Verification items for the finished model (mm, model axes). Face numbers are marked on the shaded views. Coordinates: 2 decimals unless noted, no trailing zeros. Write each loop counter-clockwise with the first axis right and the second up, starting at its lowest first coordinate (ties: lowest second). Pieces come first, ordered by that corner, then holes. Notation, with made-up numbers: (-1.5, -3.75) -> (2.5, -3.75) arc R20 ccw to (2.5, 22.25) -> close; hole circle Ø8 at (-40, 37). An arc over 180 degrees is marked (long way). Use CSV: the item, a comma, the result in double quotes.
```python
from build123d import *

# Parameters (mm, degrees)
SKETCH1_R                    = 24
SKETCH1_R_2                  = 22.8
BOSS_EXTRUDE1_DEPTH          = 2.5
BOSS_EXTRUDE5_START          = -2.5
BOSS_EXTRUDE5_DEPTH          = 1.5
CIRPATTERN1_COUNT            = 4
SKETCH2_R                    = 27
BOSS_EXTRUDE2_DEPTH          = 2
SKETCH3_R                    = 7.1
CUT_EXTRUDE1_DEPTH           = 39.448016854
SKETCH4_R                    = 8.3
SKETCH4_R_2                  = 7.1
BOSS_EXTRUDE3_DEPTH          = 2.5
BOSS_EXTRUDE4_START          = -1.5
SKETCH5_R                    = 8.3
SKETCH5_R_2                  = 6.3
BOSS_EXTRUDE4_DEPTH          = 1.5
CUT_EXTRUDE2_DEPTH           = 2.5
CHAMFER2_SIZE                = 2.5
CIRPATTERN2_COUNT            = 4
CHAMFER2_OF_CIRPATTERN2_SIZE = 2.5
FILLET1_R                    = 2
CHAMFER1_SIZE                = 0.5


# Some blends are built 0.0001 mm under size
with BuildPart() as part:
    # Sketch1 → Boss-Extrude1 (new body)
    with BuildSketch(Plane.XY):
        Circle(SKETCH1_R)
        Circle(SKETCH1_R_2, mode=Mode.SUBTRACT)
    extrude(amount=BOSS_EXTRUDE1_DEPTH)

    # Sketch6 → Boss-Extrude5 (add)
    with BuildSketch(Plane.XY.offset(2.5).offset(BOSS_EXTRUDE5_START)):
        with BuildLine():
            ThreePointArc((23.953079134, 1.5), (24, 0), (23.953079134, -1.5))
            ThreePointArc((23.953079134, -1.5), (24.3, 0), (23.953079134, 1.5))
        make_face()
    boss_extrude5 = extrude(amount=BOSS_EXTRUDE5_DEPTH)

    # CirPattern1: Boss-Extrude5 ×4 about axis
    cirpattern1_axis = Axis((0, 0, 0), (0, 0, 1))
    for i in range(1, CIRPATTERN1_COUNT):
        add(boss_extrude5.rotate(cirpattern1_axis, i * 360 / CIRPATTERN1_COUNT))

    # Sketch2 → Boss-Extrude2 (add)
    with BuildSketch(Plane.XY.offset(2.5)):
        Circle(SKETCH2_R)
    extrude(amount=BOSS_EXTRUDE2_DEPTH)

    # Sketch3 → Cut-Extrude1 (cut, through all)
    with BuildSketch(Plane.XY.offset(4.5)):
        Circle(SKETCH3_R)
    extrude(amount=-CUT_EXTRUDE1_DEPTH, mode=Mode.SUBTRACT)

    # Sketch4 → Boss-Extrude3 (add, through all)
    with BuildSketch(Plane(origin=(0, 0, 2.5), x_dir=(-1, 0, 0), z_dir=(0, 0, -1))):
        with Locations(Location((0, 0, 0), (0, 0, 180))):
            Circle(SKETCH4_R)
        with Locations(Location((0, 0, 0), (0, 0, 180))):
            Circle(SKETCH4_R_2, mode=Mode.SUBTRACT)
    extrude(amount=BOSS_EXTRUDE3_DEPTH)

    # Sketch5 → Boss-Extrude4 (add)
    with BuildSketch(Plane(origin=(0, 0, 0), x_dir=(-1, 0, 0), z_dir=(0, 0, -1)).offset(BOSS_EXTRUDE4_START)):
        with Locations(Location((0, 0, 0), (0, 0, 180))):
            Circle(SKETCH5_R)
        Circle(SKETCH5_R_2, mode=Mode.SUBTRACT)
    extrude(amount=BOSS_EXTRUDE4_DEPTH)

    # Sketch7 → Cut-Extrude2 (cut)
    with BuildSketch(Plane(origin=(0, 0, 0), x_dir=(-1, 0, 0), z_dir=(0, 0, -1))):
        with BuildLine():
            ThreePointArc((8.725182258, 21.064453341), (12.667001313, 18.95750716), (16.122034611, 16.122034611))
            Line((16.122034611, 16.122034611), (16.970562748, 16.970562748))
            ThreePointArc((16.970562748, 16.970562748), (13.333685592, 19.955270695), (9.184402377, 22.17310878))
            Line((9.184402377, 22.17310878), (8.725182258, 21.064453341))
        make_face()
        with BuildLine():
            Line((16.970562748, 16.970562748), (16.122034611, 16.122034611))
            ThreePointArc((16.122034611, 16.122034611), (18.95750716, 12.667001313), (21.064453341, 8.725182258))
            Line((21.064453341, 8.725182258), (22.17310878, 9.184402377))
            ThreePointArc((22.17310878, 9.184402377), (19.955270695, 13.333685592), (16.970562748, 16.970562748))
        make_face()
    cut_extrude2 = extrude(amount=-CUT_EXTRUDE2_DEPTH, mode=Mode.SUBTRACT)

    # Chamfer2
    chamfer2_edges = [part.edges().sort_by_distance(p)[0] for p in [
        (-21.618781061, 8.954792317, 2.5),
        (-8.954792317, 21.618781061, 2.5),
    ]]
    chamfer(chamfer2_edges, length=CHAMFER2_SIZE - 0.0001)  # a hair under: the kernel refuses the full size

    # CirPattern2: Cut-Extrude2 ×4 about axis
    cirpattern2_axis = Axis((0, 0, 0), (0, 0, 1))
    for i in range(1, CIRPATTERN2_COUNT):
        add(cut_extrude2.rotate(cirpattern2_axis, i * 360 / CIRPATTERN2_COUNT), mode=Mode.SUBTRACT)

    # Chamfer2 of CirPattern2
    chamfer2_of_cirpattern2_edges = [part.edges().sort_by_distance(p)[0] for p in [
        (-8.954792317, -21.618781061, 2.5),
        (-21.618781061, -8.954792317, 2.5),
        (21.618781061, -8.954792317, 2.5),
        (8.954792317, -21.618781061, 2.5),
        (8.954792317, 21.618781061, 2.5),
        (21.618781061, 8.954792317, 2.5),
    ]]
    chamfer(chamfer2_of_cirpattern2_edges, length=CHAMFER2_OF_CIRPATTERN2_SIZE - 0.0001)  # a hair under: the kernel refuses the full size

    # Fillet1
    # the kernel refuses this fillet: 2 mm, written as the material it adds along each edge
    with BuildSketch(Plane(origin=(0, 0, 2.5), x_dir=(1, 0, 0), z_dir=(0, 1, 0))) as fillet1_piece_1:
        with BuildLine():
            CenterArc((8.3 + FILLET1_R, FILLET1_R), FILLET1_R, 180, 90)
            Line((8.3, FILLET1_R), (8.3, 0))
            Line((8.3, 0), (8.3 + FILLET1_R, 0))
        make_face()
    revolve(axis=Axis((0, 0, 2.5), (0, 0, -1)))
    with BuildSketch(Plane(origin=(0, 0, 2.5), x_dir=(0.6608111736340745, -0.7505521919229581, 0), z_dir=(0.7505521919229581, 0.6608111736340745, 0))) as fillet1_piece_2_section:
        with BuildLine():
            CenterArc((22.8 - FILLET1_R, FILLET1_R), FILLET1_R, 270, 90)
            Line((22.8, FILLET1_R), (22.8, 0))
            Line((22.8, 0), (22.8 - FILLET1_R, 0))
        make_face()
    fillet1_piece_2 = revolve(axis=Axis((0, 0, 2.5), (0, 0, -1)), revolution_arc=82.723533759, mode=Mode.PRIVATE)
    fillet1_piece_2 = split(fillet1_piece_2, bisect_by=Plane(origin=(-4.823831946, -20.235955974, -3.287225486), z_dir=(0.653281482438186, -0.27059805007310406, 0.7071067811865476)), keep=Keep.TOP, mode=Mode.PRIVATE)
    fillet1_piece_2 = split(fillet1_piece_2, bisect_by=Plane(origin=(4.823831946, -20.235955974, -3.287225486), z_dir=(-0.6532814824381898, -0.2705980500730944, 0.7071067811865478)), keep=Keep.TOP, mode=Mode.PRIVATE)
    add(fillet1_piece_2)
    with BuildSketch(Plane(origin=(0, 0, 2.5), x_dir=(0.7505521919229583, 0.6608111736340745, 0), z_dir=(-0.6608111736340745, 0.7505521919229583, 0))) as fillet1_piece_3_section:
        with BuildLine():
            CenterArc((22.8 - FILLET1_R, FILLET1_R), FILLET1_R, 270, 90)
            Line((22.8, FILLET1_R), (22.8, 0))
            Line((22.8, 0), (22.8 - FILLET1_R, 0))
        make_face()
    fillet1_piece_3 = revolve(axis=Axis((0, 0, 2.5), (0, 0, -1)), revolution_arc=82.723533759, mode=Mode.PRIVATE)
    fillet1_piece_3 = split(fillet1_piece_3, bisect_by=Plane(origin=(20.235955974, -4.823831946, -3.287225486), z_dir=(0.2705980500731041, 0.6532814824381858, 0.7071067811865477)), keep=Keep.TOP, mode=Mode.PRIVATE)
    fillet1_piece_3 = split(fillet1_piece_3, bisect_by=Plane(origin=(20.235955974, 4.823831946, -3.287225486), z_dir=(0.27059805007309445, -0.6532814824381898, 0.7071067811865478)), keep=Keep.TOP, mode=Mode.PRIVATE)
    add(fillet1_piece_3)
    with BuildSketch(Plane(origin=(0, 0, 2.5), x_dir=(-0.750552191922958, -0.6608111736340746, 0), z_dir=(0.6608111736340746, -0.750552191922958, 0))) as fillet1_piece_4_section:
        with BuildLine():
            CenterArc((22.8 - FILLET1_R, FILLET1_R), FILLET1_R, 270, 90)
            Line((22.8, FILLET1_R), (22.8, 0))
            Line((22.8, 0), (22.8 - FILLET1_R, 0))
        make_face()
    fillet1_piece_4 = revolve(axis=Axis((0, 0, 2.5), (0, 0, -1)), revolution_arc=82.723533759, mode=Mode.PRIVATE)
    fillet1_piece_4 = split(fillet1_piece_4, bisect_by=Plane(origin=(-20.235955974, 4.823831946, -3.287225486), z_dir=(-0.2705980500731042, -0.6532814824381858, 0.7071067811865477)), keep=Keep.TOP, mode=Mode.PRIVATE)
    fillet1_piece_4 = split(fillet1_piece_4, bisect_by=Plane(origin=(-20.235955974, -4.823831946, -3.287225486), z_dir=(-0.2705980500730945, 0.6532814824381897, 0.7071067811865478)), keep=Keep.TOP, mode=Mode.PRIVATE)
    add(fillet1_piece_4)
    with BuildSketch(Plane(origin=(0, 0, 2.5), x_dir=(-0.6608111736340749, 0.7505521919229577, 0), z_dir=(-0.7505521919229577, -0.6608111736340749, 0))) as fillet1_piece_5_section:
        with BuildLine():
            CenterArc((22.8 - FILLET1_R, FILLET1_R), FILLET1_R, 270, 90)
            Line((22.8, FILLET1_R), (22.8, 0))
            Line((22.8, 0), (22.8 - FILLET1_R, 0))
        make_face()
    fillet1_piece_5 = revolve(axis=Axis((0, 0, 2.5), (0, 0, -1)), revolution_arc=82.723533759, mode=Mode.PRIVATE)
    fillet1_piece_5 = split(fillet1_piece_5, bisect_by=Plane(origin=(-4.823831946, 20.235955974, -3.287225486), z_dir=(0.6532814824381898, 0.2705980500730944, 0.7071067811865478)), keep=Keep.TOP, mode=Mode.PRIVATE)
    fillet1_piece_5 = split(fillet1_piece_5, bisect_by=Plane(origin=(4.823831946, 20.235955974, -3.287225486), z_dir=(-0.6532814824381858, 0.2705980500731041, 0.7071067811865477)), keep=Keep.TOP, mode=Mode.PRIVATE)
    add(fillet1_piece_5)

    # Chamfer1
    chamfer1_edges = [part.edges().sort_by_distance(p)[0] for p in [
        (-27, 0, 4.5),
        (-7.1, 0, 4.5),
    ]]
    chamfer(chamfer1_edges, length=CHAMFER1_SIZE)


solid = part.part
```
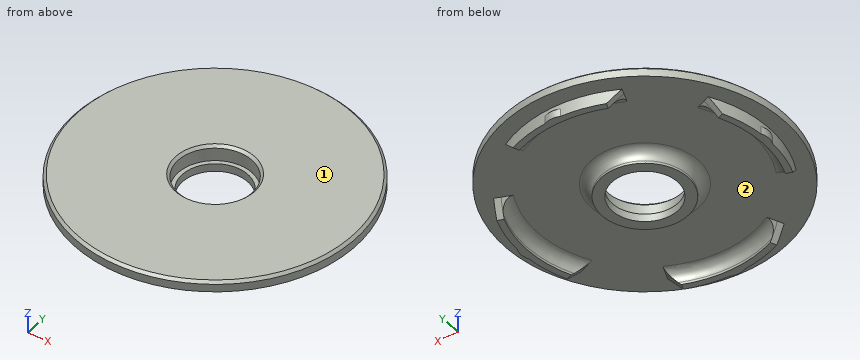
1) Scan lines: L1, parallel to Y at x = 0, z = 0.4; L2, parallel to Y at x = 0, z = 3.15; L3, parallel to Z at x = 16, y = -11.5. Record each from-to range of solid material in increasing order.
Return value:
L1,"-24.3 to -22.8, -8.3 to -6.3, 6.3 to 8.3, 22.8 to 24.3"
L2,"-27 to -7.1, 7.1 to 27"
L3,"2.5 to 4.5"
2) Cross-section at A-A (z = 3.15). Record the boundary of the cut face in (x, y).
Return value:
outline,"circle Ø54 at (0, 0); hole circle Ø14.2 at (0, 0)"
3) Gauge pin test, flat ends, axial feed: pin 1 (3 mm diameter, centred on x = -13, y = 12.5, fed in from -Z); pin 2 (7 mm diameter, centred on x = 1, y = 3, fed in from +Z); pin 3 (1 mm diameter, centred on y = 8, z = 3.5, fed in from +X). Record the tip position at first contact, or that the pin passes through.
Return value:
pin 1,"z = 2.5"
pin 2,"z = 1.5"
pin 3,"x = 25.94"
4) Mould release check, pull along Y, two halves, no side actions. Record for the marked faces 1 and 2: released by +Y, released by -Y, zero draft, split by the parting line, or undercut.
Return value:
face 1,"zero draft"
face 2,"undercut"
